from build123d import *

# Parameters (mm, degrees)
SKETCH2_R           = 5
BOSS_EXTRUDE1_DEPTH = 7
BOSS_EXTRUDE2_DEPTH = 12.5
BOSS_EXTRUDE3_DEPTH = 0.2
SKETCH5_R           = 2
BOSS_EXTRUDE4_DEPTH = 1
SKETCH6_R           = 0.5
CUT_EXTRUDE1_DEPTH  = 2
SKETCH7_R           = 0.45
BOSS_EXTRUDE5_DEPTH = 6
SKETCH8_R           = 3.5
BOSS_EXTRUDE6_DEPTH = 0.02
SKETCH9_R           = 2.675
BOSS_EXTRUDE7_DEPTH = 3.1
SKETCH10_R          = 1.675
CUT_EXTRUDE2_DEPTH  = 2


with BuildPart() as part:
    # Sketch2 → Boss-Extrude1 (new body)
    with BuildSketch(Plane(origin=(0, 0, 0), x_dir=(1, 0, 0), z_dir=(0, 1, 0))):
        with Locations(Location((0, 0, 0), (0, 0, 270))):
            Circle(SKETCH2_R)
    extrude(amount=BOSS_EXTRUDE1_DEPTH)

    # Sketch3 → Boss-Extrude2 (add)
    with BuildSketch(Plane(origin=(0, 7, 0), x_dir=(1, 0, 0), z_dir=(0, 1, 0))):
        with BuildLine():
            Line((-3.975, 2.99165506), (-3.975, -2.99165506))
            ThreePointArc((-3.975, -2.99165506), (0, -4.975), (3.975, -2.99165506))
            Line((3.975, -2.99165506), (3.975, 2.99165506))
            ThreePointArc((3.975, 2.99165506), (0, 4.975), (-3.975, 2.99165506))
        make_face()
    extrude(amount=BOSS_EXTRUDE2_DEPTH)

    # Sketch4 → Boss-Extrude3 (add)
    with BuildSketch(Plane(origin=(0, 19.5, 0), x_dir=(1, 0, 0), z_dir=(0, 1, 0))):
        with BuildLine():
            Line((-3.2, 3.5), (-2.1, 3.5))
            ThreePointArc((-2.1, 3.5), (-1.569669914, 3.280330086), (-1.35, 2.75))
            Line((-1.35, 2.75), (-1.35, -5))
            Line((-1.35, -5), (-3.95, -5))
            Line((-3.95, -5), (-3.95, 2.75))
            ThreePointArc((-3.95, 2.75), (-3.730330086, 3.280330086), (-3.2, 3.5))
        make_face()
        with BuildLine():
            Line((3.95, -5), (1.35, -5))
            Line((1.35, -5), (1.35, 2.75))
            ThreePointArc((1.35, 2.75), (1.569669914, 3.280330086), (2.1, 3.5))
            Line((2.1, 3.5), (3.2, 3.5))
            ThreePointArc((3.2, 3.5), (3.730330086, 3.280330086), (3.95, 2.75))
            Line((3.95, 2.75), (3.95, -5))
        make_face()
    extrude(amount=BOSS_EXTRUDE3_DEPTH)

    # Sketch5 → Boss-Extrude4 (add)
    with BuildSketch(Plane(origin=(0, 19.5, 0), x_dir=(1, 0, 0), z_dir=(0, 1, 0))):
        with Locations(Location((0, 0, 0), (0, 0, 47.545849796))):
            Circle(SKETCH5_R)
    extrude(amount=BOSS_EXTRUDE4_DEPTH)

    # Sketch6 → Cut-Extrude1 (cut)
    with BuildSketch(Plane(origin=(0, 20.5, 0), x_dir=(1, 0, 0), z_dir=(0, 1, 0))):
        with Locations(Location((0, 0, 0), (0, 0, 270))):
            Circle(SKETCH6_R)
    extrude(amount=-CUT_EXTRUDE1_DEPTH, mode=Mode.SUBTRACT)

    # Sketch7 → Boss-Extrude5 (add)
    with BuildSketch(Plane(origin=(0, 18.5, 0), x_dir=(1, 0, 0), z_dir=(0, 1, 0))):
        with Locations(Location((0, 0, 0), (0, 0, 270))):
            Circle(SKETCH7_R)
    extrude(amount=BOSS_EXTRUDE5_DEPTH)

    # Sketch8 → Boss-Extrude6 (add)
    with BuildSketch(Plane.XZ):
        with Locations(Location((0, 0, 0), (0, 0, 90))):
            Circle(SKETCH8_R)
    extrude(amount=BOSS_EXTRUDE6_DEPTH)

    # Sketch9 → Boss-Extrude7 (add)
    with BuildSketch(Plane.XZ.offset(0.02)):
        with Locations(Location((0, 0, 0), (0, 0, 90))):
            Circle(SKETCH9_R)
    extrude(amount=BOSS_EXTRUDE7_DEPTH)

    # Sketch10 → Cut-Extrude2 (cut)
    with BuildSketch(Plane.XZ.offset(3.12)):
        with Locations(Location((0, 0, 0), (0, 0, 270))):
            Circle(SKETCH10_R)
    extrude(amount=-CUT_EXTRUDE2_DEPTH, mode=Mode.SUBTRACT)


solid = part.part
Build history of the part. All positions in model axes, mm. A direction names the side the tool comes from. Round coordinates to 2 decimals unless told otherwise and drop trailing zeros. Loops run counter-clockwise (first coordinate to the right, second up) from the corner with the lowest first, then second, coordinate; pieces in that order, holes last. Notation, with made-up numbers: (47.5, 44.5) -> (53.5, 44.5) arc R13 cw to (53.5, 68.5) -> close; hole circle Ø9 at (33.5, -17). An arc over 180 degrees is marked (long way). Answer in a Markdown table with one row per item.
Item 1: Saw through at B-B (y = 5.25). Write the cut outline in (x, z).
Answers below:
| item | result |
|---|---|
| outline | circle Ø10 at (0, 0) |
Item 2: Drill centre lines: L1, parallel to Y at x = 3.25, z = -1.75; L2, parallel to X at y = -2.6, z = 0 (3 decimals); L3, parallel to X at y = 12.5, z = -2 (3 decimals). Where is each one in solid material? Low to high. Write a range as [from, to].
Answers below:
| item | result |
|---|---|
| L1 | y = [0, 19.7] |
| L2 | x = [-2.675, -1.675], [1.675, 2.675] |
| L3 | x = [-3.975, 3.975] |
Item 3: Which spindle directions (+Z, -Z, +X, -X, +Y, -Y) get a long thin tool onto all of the face, cutting with end or side? Do faces 5 (the cylindrical face through (0.064, 13.162, -4.975)), 6 (the cylindrical face through (-0.064, 13.162, 4.975)), 7 (the flat face through (0, 19.5, 3)), 8 (the flat face through (-3.3, 0, 2.2)). Say none if no direction does.
Answers below:
| item | result |
|---|---|
| face 5 | -Z, +Y |
| face 6 | +Z |
| face 7 | +Z, +Y |
| face 8 | -Y |
Item 4: Pin check, flat tips, straight feed: pin 1 (2 mm diameter, centred on x = -2.5, y = 6.5, fed in from +Z); pin 2 (3 mm diameter, centred on x = 2.5, z = -0.5, fed in from +Y); pin 3 (4.5 mm diameter, centred on x = -0.5, z = 0, fed in from +Y); pin 4 (5 mm diameter, centred on x = -3.5, y = 12, fed in from +Z). Stop position of each tip, or through.
Answers below:
| item | result |
|---|---|
| pin 1 | stops at z = 4.77 |
| pin 2 | stops at y = 20.5 |
| pin 3 | stops at y = 24.5 |
| pin 4 | stops at z = 4.87 |
Item 5: Mould opens along X. For faces 1 (the flat face through (3.975, 13, 0)), 2 (the flat face through (0, 24.5, 0)), 3 (the cylindrical face through (-4.88, 3.45, -1.08)), 4 (the cylindrical face through (-0.172, 21.458, 0.416)) say: +X half, -X half, draft (parallel to the pull), parting line (faces both ways), or undercut.
Answers below:
| item | result |
|---|---|
| face 1 | +X half |
| face 2 | draft |
| face 3 | parting line |
| face 4 | undercut |
